Check sheet for the modelled part. Datum: model origin and axes. Units: mm. A direction names the side the tool comes from. Round coordinates to 2 decimals unless told otherwise and drop trailing zeros. Loops run counter-clockwise (first coordinate to the right, second up) from the corner with the lowest first, then second, coordinate; pieces in that order, holes last. Notation, with made-up numbers: (85.25, 39.25) -> (104.25, 39.25) arc R21 ccw to (104.25, 47.25) -> close; hole circle Ø3 at (-26.5, 82.5). An arc over 180 degrees is marked (long way). Return JSON: item names as keys, results as strings.
from build123d import *

# Parameters (mm, degrees)
SKETCH_1_W             = 34
SKETCH_1_H             = 37.5
EXTRUDE_282_DEPTH      = 44.5
SKETCH_2_W             = 12
SKETCH_2_H             = 37.5
EXTRUDE_458_DEPTH      = 1
SKETCH_3_R             = 6.5
CUT_EXTRUDE_1_DEPTH    = 61.625902055
SKETCH_4_R             = 11
CUT_EXTRUDE_843_DEPTH  = 13
CUT_EXTRUDE_START      = -14
SKETCH_5_R             = 11
CUT_EXTRUDE_1029_DEPTH = 14


with BuildPart() as part:
    # Эскиз1 → Extrude 282 (new body)
    with BuildSketch(Plane(origin=(0, 0, 0), x_dir=(1, 0, 0), z_dir=(0, 1, 0))):
        Rectangle(SKETCH_1_W, SKETCH_1_H)
    extrude(amount=EXTRUDE_282_DEPTH)

    # Эскиз2 → Extrude 458 (add)
    with BuildSketch(Plane.XZ):
        Rectangle(SKETCH_2_W, SKETCH_2_H)
    extrude(amount=EXTRUDE_458_DEPTH)

    # Эскиз3 → Вырез-Вытянуть1 (cut, through all)
    with BuildSketch(Plane.XY.offset(18.75)):
        with Locations((0, 26.5)):
            Circle(SKETCH_3_R)
    extrude(amount=-CUT_EXTRUDE_1_DEPTH, mode=Mode.SUBTRACT)

    # Эскиз4 → Cut-Extrude 843 (cut)
    with BuildSketch(Plane.XY.offset(18.75)):
        with Locations((0, 26.5)):
            Circle(SKETCH_4_R)
    extrude(amount=-CUT_EXTRUDE_843_DEPTH, mode=Mode.SUBTRACT)

    # Эскиз5 → Cut-Extrude 1029 (cut)
    with BuildSketch(Plane(origin=(0, 0, -18.75), x_dir=(-1, 0, 0), z_dir=(0, 0, -1)).offset(CUT_EXTRUDE_START)):
        with Locations(Location((0, 26.5, 0), (0, 0, 180))):
            Circle(SKETCH_5_R)
    extrude(amount=CUT_EXTRUDE_1029_DEPTH, mode=Mode.SUBTRACT)

    # Эскиз7 → К профилю M6 (revolve, cut)
    with BuildSketch(Plane(origin=(0, 44.5, 0), x_dir=(0, 0, 1), z_dir=(1, 0, 0))):
        Polygon((0, 0), (0, 45.5), (3.3, 45.5), (3.3, 35.6), (8, 35.6), (8, 0.025), (8.025, 0), align=None)
    revolve(axis=Axis((0, 50.85, 0), (0, -1, 0)), mode=Mode.SUBTRACT)


solid = part.part
Q1. Section check B-B (y = 26.5). Record the boundary of the cut face in (x, z).
Results list:
{"outline": "(-17, -18.75) -> (-11, -18.75) -> (-11, -4.75) -> (-6.5, -4.75) -> (-6.5, -4.66) arc R8 cw to (-6.5, 4.66) -> (-6.5, 5.75) -> (-11, 5.75) -> (-11, 18.75) -> (-17, 18.75) -> close; (6.5, -4.75) -> (11, -4.75) -> (11, -18.75) -> (17, -18.75) -> (17, 18.75) -> (11, 18.75) -> (11, 5.75) -> (6.5, 5.75) -> (6.5, 4.66) arc R8 cw to (6.5, -4.66) -> close"}
Q2. Tool access check on faces 1 (the cylindrical face through (10.161, 22.287, 12.341)), 2 (the flat face through (8, 26, -4.75)), 3 (the cylindrical face through (7.1, 26.94, 3.69)), 4 (the cylindrical face through (6.5, 26.5, 5.3)). Record the directions out of +Z, -Z, +X, -X, +Y, -Y that give a thin tool (end or side, any length) a straight path to the whole face; none if there is none.
Results list:
{"face 1": "+Z", "face 2": "-Z", "face 3": "+Y", "face 4": "+Z, -Z"}
Q3. Draft check along Z on faces 5 (the flat face through (7, 16, -18.75)), 6 (the flat face through (2, 8.9, -3)), 7 (the flat face through (0, 44.5, -9)). Enter one of: released by +Z, released by -Z, zero draft, split by the parting line, or undercut.
Results list:
{"face 5": "released by -Z", "face 6": "undercut", "face 7": "zero draft"}
Q4. Section check D-D (x = 0). Record the boundary of the cut face in (y, z) (3 decimals).
Results list:
{"outline": "(-1, -18.75) -> (15.5, -18.75) -> (15.5, -8) -> (8.9, -8) -> (8.9, -3.3) -> (-1, -3.3) -> close; (-1, 3.3) -> (8.9, 3.3) -> (8.9, 8) -> (15.5, 8) -> (15.5, 18.75) -> (-1, 18.75) -> close; (37.5, -18.75) -> (44.5, -18.75) -> (44.5, -8.025) -> (44.475, -8) -> (37.5, -8) -> close; (37.5, 8) -> (44.475, 8) -> (44.5, 8.025) -> (44.5, 18.75) -> (37.5, 18.75) -> close"}
Q5. Material ranges on line 1 (X direction, y = 7.25, z = 0); line 2 (X direction, y = 26.5, z = -8); line 3 (Z direction, x = 0, y = 5), recorded low to high.
Results list:
{"line 1": "-17 to -3.3, 3.3 to 17", "line 2": "-17 to -11, 11 to 17", "line 3": "-18.75 to -3.3, 3.3 to 18.75"}
Q6. Section check A-A (z = 0). Record the boundary of the cut face in (x, y) (3 decimals), then the cut area to 3 significant figures.
Results list:
{"outline": "(-17, 0) -> (-6, 0) -> (-6, -1) -> (-3.3, -1) -> (-3.3, 8.9) -> (-8, 8.9) -> (-8, 44.475) -> (-8.025, 44.5) -> (-17, 44.5) -> close; (3.3, -1) -> (6, -1) -> (6, 0) -> (17, 0) -> (17, 44.5) -> (8.025, 44.5) -> (8, 44.475) -> (8, 8.9) -> (3.3, 8.9) -> close", "area": "890 mm^2"}
Q7. Section check C-C (z = -15.5). Record the boundary of the cut face in (x, y).
Results list:
{"outline": "(-17, 0) -> (-6, 0) -> (-6, -1) -> (6, -1) -> (6, 0) -> (17, 0) -> (17, 44.5) -> (-17, 44.5) -> close; hole circle Ø22 at (0, 26.5)"}
Q8. Go/stop test with flat-tipped pins: pin 1 (1.6 mm diameter, centred on x = 9, y = 22, fed in from +Z); pin 2 (8 mm diameter, centred on x = 0.5, z = -1, fed in from +Y); pin 3 (9 mm diameter, centred on x = -11.5, z = 4.5, fed in from -Y). Record where each tip stops, or that it passes through.
Results list:
{"pin 1": "z = 5.75", "pin 2": "y = 8.9", "pin 3": "y = 0"}
